```python
from build123d import *

# Parameters (mm, degrees)
F0_W     = 90
F0_H     = 40
F1_DEPTH = 8
F2_SIZE  = 2.5
F4_D     = 4.4
F5_D     = 4.4
F6_D     = 18.5
F7_D     = 12
F8_D     = 5.5


with BuildPart() as f1:
    # F0 (on Front) → F1 (new body)
    with BuildSketch(Plane.XZ):
        Rectangle(F0_W, F0_H)
    extrude(amount=F1_DEPTH)

    # F2
    f2_edges = [f1.edges().sort_by_distance(p)[0] for p in [
        (-45, -4, -20),
        (45, -4, -20),
    ]]
    chamfer(f2_edges, length=F2_SIZE)

    # F4 (through all)
    with Locations(Plane.XZ.offset(8)):
        with Locations((-36, 16), (-12, 16), (12, 16), (36, 16)):
            Hole(F4_D / 2)

    # F5 (through all)
    with Locations(Plane.XZ.offset(8)):
        with Locations((-40.313708499, 11.313708499), (-17.686291501, 11.313708499), (-17.686291501, -11.313708499), (-40.313708499, -11.313708499), (17.686291501, 11.313708499), (40.313708499, 11.313708499), (40.313708499, -11.313708499), (17.686291501, -11.313708499)):
            Hole(F5_D / 2)

    # F6 (through all)
    with Locations(Plane.XZ.offset(8)):
        with Locations((-29, 0), (29, 0)):
            Hole(F6_D / 2)

    # F7 (through all)
    with Locations(Plane.XZ.offset(8)):
        with Locations((0, -5)):
            Hole(F7_D / 2)

    # F8 (through all)
    with Locations(Plane.XZ.offset(8)):
        with Locations((7, -12), (-7, 2), (7, 2), (-7, -12)):
            Hole(F8_D / 2)


solid = f1.part
```
Input: part model. Units: mm. Frame: model coordinates. Give positions to 0.01 mm unless a question says otherwise; leave off trailing zeros. Write each loop counter-clockwise with the first axis right and the second up, starting at its lowest first coordinate (ties: lowest second). Pieces come first, ordered by that corner, then holes. Notation, with made-up numbers: (-23.75, 58) - (1.25, 58) arc R11 ccw to (1.25, 78) - close; hole circle Ø10 at (-25.5, 14.25). An arc over 180 degrees is marked (long way). Write item = value, one per line. Start each with the question number.
1) Pin query (flat end, axial travel): pin 1 (14 mm diameter, centred on x = 0, z = -5, fed in from +Y); pin 2 (15 mm diameter, centred on x = -29, z = 0, fed in from +Y). Return the tip coordinate at first contact, or that it passes through.
2) Cut plane A-A (x = 7). Return loops of the section in (y, z), and give its area (3 significant figures).
3) Draft query along X for faces 1 (the face through (-43.7, -3.9, -18.8)), 2 (the face through (38.3, -3.9, -12.2)), 3 (the face through (-1, -4, -20)). Return one class per face: pulls with the +X half, pulls with the -X half, needs draft (parallel to the pull), parting line crosses it, or undercut.
4) Cut plane C-C (x = -12). Return loops of the section in (y, z).
5) Cut plane B-B (z = 16). Return loops of the section in (x, y).
6) Cut plane D-D (z = -5). Return loops of the section in (x, y).
7) Material intervals for L1, parallel to X at y = -3.5, z = 14.5; L2, parallel to Z at x = 29.5, y = -1.25; L3, parallel to X at y = -5.25, z = 12, sorted ascending. Write a range as [from, to].
Answers follow:
q1.pin_1 = 0
q1.pin_2 = through
q2.outline = (-8, -20) - (0, -20) - (0, -14.75) - (-8, -14.75) - close; (-8, -9.25) - (0, -9.25) - (0, -0.75) - (-8, -0.75) - close; (-8, 4.75) - (0, 4.75) - (0, 20) - (-8, 20) - close
q2.area = 232 mm^2
q3.face_1 = pulls with the -X half
q3.face_2 = undercut
q3.face_3 = needs draft
q4.outline = (-8, -20) - (0, -20) - (0, 13.8) - (-8, 13.8) - close; (-8, 18.2) - (0, 18.2) - (0, 20) - (-8, 20) - close
q5.outline = (-45, -8) - (-38.2, -8) - (-38.2, 0) - (-45, 0) - close; (-33.8, -8) - (-14.2, -8) - (-14.2, 0) - (-33.8, 0) - close; (-9.8, -8) - (9.8, -8) - (9.8, 0) - (-9.8, 0) - close; (14.2, -8) - (33.8, -8) - (33.8, 0) - (14.2, 0) - close; (38.2, -8) - (45, -8) - (45, 0) - (38.2, 0) - close
q6.outline = (-45, -8) - (-36.78, -8) - (-36.78, 0) - (-45, 0) - close; (-21.22, -8) - (-6, -8) - (-6, 0) - (-21.22, 0) - close; (6, -8) - (21.22, -8) - (21.22, 0) - (6, 0) - close; (36.78, -8) - (45, -8) - (45, 0) - (36.78, 0) - close
q7.L1 = [-45, -37.61], [-34.39, -13.61], [-10.39, 10.39], [13.61, 34.39], [37.61, 45]
q7.L2 = [-20, -9.24], [9.24, 20]
q7.L3 = [-45, -42.4], [-38.22, -19.78], [-15.6, 15.6], [19.78, 38.22], [42.4, 45]
